from build123d import *

# Parameters (mm, degrees)
SKETCH2_W                       = 38.1
SKETCH2_H                       = 6.35
BOSS_EXTRUDE1_DEPTH             = 152.4
CBORE_FOR_M3_SBHCS1_D           = 3.4
CBORE_FOR_M3_SBHCS1_CBORE_D     = 6.7
CBORE_FOR_M3_SBHCS1_CBORE_DEPTH = 1.65
SKETCH9_W                       = 3.048
SKETCH9_H                       = 3.048
CUT_EXTRUDE1_DEPTH              = 5.588
SKETCH12_W                      = 128.27
SKETCH12_H                      = 5.08
CUT_EXTRUDE2_DEPTH              = 3.048
SKETCH13_W                      = 18.542
SKETCH13_H                      = 1.905
CUT_EXTRUDE3_DEPTH              = 3.048
CUT_EXTRUDE4_DEPTH              = 6.35
CUT_EXTRUDE5_DEPTH              = 6.35
CUT_EXTRUDE7_DEPTH              = 154.618824123
CUT_EXTRUDE7_DEPTH_BACK         = 59.944
SKETCH19_W                      = 38.1
SKETCH19_H                      = 2.032
CUT_EXTRUDE9_DEPTH              = 92.456


with BuildPart() as part:
    # Sketch2 → Boss-Extrude1 (new body)
    with BuildSketch(Plane(origin=(0, 0, 0), x_dir=(0, 0, -1), z_dir=(1, 0, 0))):
        Rectangle(SKETCH2_W, SKETCH2_H)
    extrude(amount=BOSS_EXTRUDE1_DEPTH)

    # CBORE for M3 SBHCS1 (through all)
    with Locations(Plane(origin=(0, 3.175, 0), x_dir=(1, 0, 0), z_dir=(0, 1, 0))):
        with Locations((142.367, -7.493), (142.367, 7.493), (102.489, 7.493), (102.489, -7.493), (132.334, 10.033), (112.268, 10.032595549), (112.395401903, -10.033), (132.461, -9.906)):
            CounterBoreHole(CBORE_FOR_M3_SBHCS1_D / 2, CBORE_FOR_M3_SBHCS1_CBORE_D / 2, CBORE_FOR_M3_SBHCS1_CBORE_DEPTH)

    # Sketch9 → Cut-Extrude1 (cut)
    with BuildSketch(Plane.ZY):
        with Locations((0, 1.651)):
            Rectangle(SKETCH9_W, SKETCH9_H)
    extrude(amount=-CUT_EXTRUDE1_DEPTH, mode=Mode.SUBTRACT)

    # Sketch12 → Cut-Extrude2 (cut)
    with BuildSketch(Plane(origin=(0, 3.175, 0), x_dir=(1, 0, 0), z_dir=(0, 1, 0))):
        with Locations((88.265, 0)):
            Rectangle(SKETCH12_W, SKETCH12_H)
    extrude(amount=-CUT_EXTRUDE2_DEPTH, mode=Mode.SUBTRACT)

    # Sketch13 → Cut-Extrude3 (cut)
    with BuildSketch(Plane(origin=(0, 3.175, 0), x_dir=(1, 0, 0), z_dir=(0, 1, 0))):
        with Locations((14.859, 0.0635)):
            Rectangle(SKETCH13_W, SKETCH13_H)
    extrude(amount=-CUT_EXTRUDE3_DEPTH, mode=Mode.SUBTRACT)

    # Sketch14 → Cut-Extrude4 (cut)
    with BuildSketch(Plane(origin=(0, 3.175, 0), x_dir=(1, 0, 0), z_dir=(0, 1, 0))):
        Polygon((0, 6.35), (0, 19.05), (101.6, 19.05), align=None)
    extrude(amount=-CUT_EXTRUDE4_DEPTH, mode=Mode.SUBTRACT)

    # Sketch15 → Cut-Extrude5 (cut)
    with BuildSketch(Plane(origin=(0, 3.175, 0), x_dir=(1, 0, 0), z_dir=(0, 1, 0))):
        Polygon((0, -6.35), (101.6, -19.05), (0, -19.05), align=None)
    extrude(amount=-CUT_EXTRUDE5_DEPTH, mode=Mode.SUBTRACT)

    # Sketch17 → Cut-Extrude7 (cut, two sides: drawn at the far end of the back side and taken through both)
    with BuildSketch(Plane(origin=(152.4, 0, 0), x_dir=(0, 0, -1), z_dir=(1, 0, 0)).offset(-CUT_EXTRUDE7_DEPTH_BACK)):
        Polygon((-105.766830618, -1.27), (-19.05, -1.27), (-2.921, -1.27), (-2.921, -1.905), (-1.27, -1.905), (-1.27, -3.175), (1.524, -3.175), (1.524, -1.905), (2.921, -1.905), (2.921, -1.27), (19.05, -1.27), (105.766830618, -1.27), (105.766830618, -174.703661235), (-105.766830618, -174.703661235), align=None)
    extrude(amount=CUT_EXTRUDE7_DEPTH + CUT_EXTRUDE7_DEPTH_BACK, mode=Mode.SUBTRACT)

    # Sketch19 → Cut-Extrude9 (cut)
    with BuildSketch(Plane.ZY):
        with Locations((0, -2.286)):
            Rectangle(SKETCH19_W, SKETCH19_H)
    extrude(amount=-CUT_EXTRUDE9_DEPTH, mode=Mode.SUBTRACT)


solid = part.part
Could you check a few things on this model? Use its own coordinates, in mm. A direction names the side the tool comes from. Coordinates: 2 decimals unless noted, no trailing zeros. Order: outer loops, then holes, each group sorted by start corner. A loop starts at its lowest first (then second) coordinate and runs counter-clockwise, first axis right, second up.
Q1. Which directions (+Z, -Z, +X, -X, +Y, -Y) give clear straight access to the entire face, cutting with the end or side of a thin tool? Please do faces 5 (the flat face through (111, 1.525, -12)), 6 (the flat face through (15, 2, 0.889)), 7 (the cylindrical face through (130.84, 0.11, 9.4)), 8 (the flat face through (3, 2, -1.524)).
Q2. Suppose I cut it at D-D on x = 76. Please give me the cut outline in (y, z) (3 decimals).
Q3. Suppose I cut it at B-B on z = 17. Please give me the cut outline in (x, y) (3 decimals), and give its area (3 significant figures).
Q4. Please list where these lines run through material, in increasing order: L1, parallel to Z at x = 109, y = 1; L2, parallel to Z at x = 36, y = 0; L3, parallel to X at y = 2.25, z = -6.
Q5. Will these pins go through, and if not, where does the flat tip stop? pin 1 (2 mm diameter, centred on x = 101, z = -8, fed in from +Y) (3 decimals); pin 2 (3 mm diameter, centred on x = 52.5, y = 2.5, fed in from -Z); pin 3 (6 mm diameter, centred on x = 132.461, z = 9.906, fed in from -Y).
Q6. Thinking about a two-plate mould opening in X: for faces 1 (the flat face through (127, 1, 19.05)), 2 (the cylindrical face through (100.868, 0.108, -8.004)), 3 (the flat face through (152.4, -1, 0)), 4 (the flat face through (0, -0.5, 0.1)), which applies, released by +X, released by -X, zero draft, split by the parting line, or undercut?
Q7. Suppose I cut it at C-C on x = 58. Please give me the cut outline in (y, z) (3 decimals), and give its area (3 significant figures).
Q8. Suppose I cut it at A-A on x = 94. Please give me the cut outline in (y, z) (3 decimals).
Answer:
1. face 5: +Y
1. face 6: +X, -X, +Y
1. face 7: +Y, -Y
1. face 8: -X, +Y
2. outline: (-1.27, -15.85) - (3.175, -15.85) - (3.175, -2.54) - (0.127, -2.54) - (0.127, 2.54) - (3.175, 2.54) - (3.175, 15.85) - (-1.27, 15.85) - close
3. outline: (85.2, -1.27) - (152.4, -1.27) - (152.4, 3.175) - (85.2, 3.175) - close
3. area: 299 mm2
4. L1: z = -19.05 to -2.54, 2.54 to 19.05
4. L2: z = -10.85 to 10.85
4. L3: x = 0 to 99.49, 105.49 to 139.37, 145.37 to 152.4
5. pin 1: stops at y = 1.525
5. pin 2: stops at z = -13.1
5. pin 3: stops at y = -1.27
6. face 1: zero draft
6. face 2: undercut
6. face 3: released by +X
6. face 4: released by -X
7. outline: (-1.27, -13.6) - (3.175, -13.6) - (3.175, -2.54) - (0.127, -2.54) - (0.127, 2.54) - (3.175, 2.54) - (3.175, 13.6) - (-1.27, 13.6) - close
7. area: 105 mm2
8. outline: (-3.175, -1.524) - (-1.905, -1.524) - (-1.905, -2.921) - (-1.27, -2.921) - (-1.27, -18.1) - (3.175, -18.1) - (3.175, -2.54) - (0.127, -2.54) - (0.127, 2.54) - (3.175, 2.54) - (3.175, 18.1) - (-1.27, 18.1) - (-1.27, 2.921) - (-1.905, 2.921) - (-1.905, 1.27) - (-3.175, 1.27) - close
